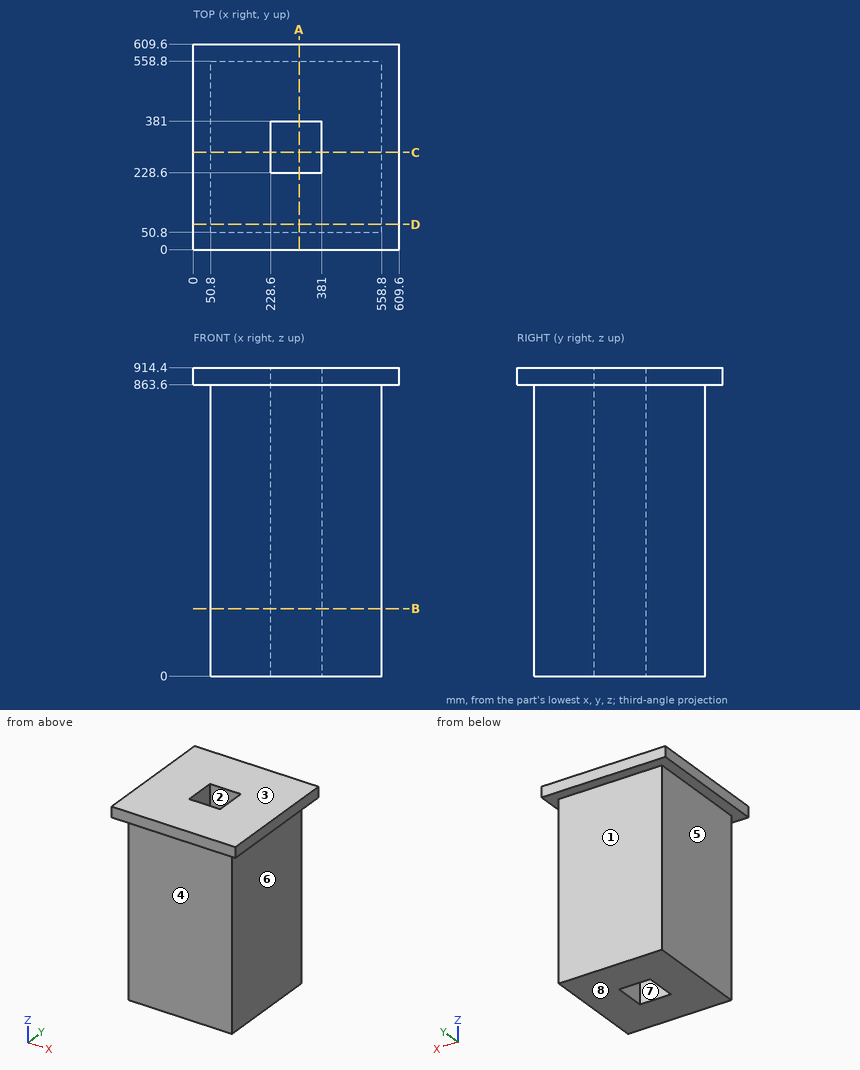
Print and shaded views of the part. All mm, measured from the part's lowest x, y and z. A direction names the side the tool comes from. Coordinates: 2 decimals unless noted, no trailing zeros. Order: outer loops, then holes, each group sorted by start corner. A loop starts at its lowest first (then second) coordinate and runs counter-clockwise, first axis right, second up. Notation, with made-up numbers: (26, 27) -> (47, 27) arc R12 cw to (47, 44) -> close; hole circle Ø8 at (6, 76). An arc over 180 degrees is marked (long way). Answer as a JSON object with one key per item and string values. Group by question number.
1) Pull direction X, two halves, no side cores. Call the marked faces 6, 7 and 8: +X half, -X half, draft (parallel to the pull), parting line (faces both ways), or undercut.
2) Flat gauge pins, fed straight in: pin 1 (3 mm diameter, centred on x = 88.5, y = 104, fed in from -Z); pin 2 (8 mm diameter, centred on y = 502, z = 176.5, fed in from +X); pin 3 (1.5 mm diameter, centred on x = 263.5, z = 226.5, fed in from +Y); pin 4 (5 mm diameter, centred on x = 315.5, z = 148, fed in from -Y). Where does each tip first touch, or does it go through?
3) Drill centre lines: L1, parallel to Y at x = 345, z = 298.5; L2, parallel to X at y = 139, z = 670. Where is each one in solid material? Low to high.
4) Cut at B-B, the plane z = 200. Write the cut outline in (x, y).
5) Cut at A-A, the plane x = 313.5. Write the cut outline in (y, z).
6) Cut at D-D, the plane y = 75. Write the cut outline in (x, z), then the cut area to 3 significant figures.
7) Which spindle directions (+Z, -Z, +X, -X, +Y, -Y) get a long thin tool onto all of the face, cutting with end or side? Do the marked faces 1, 2, 3, 4 and 5. Say none if no direction does.
Check values:
{
 "1": {"face 6": "+X half", "face 7": "undercut", "face 8": "draft"},
 "2": {"pin 1": "stops at z = 0", "pin 2": "stops at x = 558.8", "pin 3": "stops at y = 558.8", "pin 4": "stops at y = 50.8"},
 "3": {"L1": "y = 50.8 to 228.6, 381 to 558.8", "L2": "x = 50.8 to 558.8"},
 "4": {"outline": "(50.8, 50.8) -> (558.8, 50.8) -> (558.8, 558.8) -> (50.8, 558.8) -> close; hole (228.6, 228.6) -> (381, 228.6) -> (381, 381) -> (228.6, 381) -> close"},
 "5": {"outline": "(0, 863.6) -> (50.8, 863.6) -> (50.8, 0) -> (228.6, 0) -> (228.6, 914.4) -> (0, 914.4) -> close; (381, 0) -> (558.8, 0) -> (558.8, 863.6) -> (609.6, 863.6) -> (609.6, 914.4) -> (381, 914.4) -> close"},
 "6": {"outline": "(0, 863.6) -> (50.8, 863.6) -> (50.8, 0) -> (558.8, 0) -> (558.8, 863.6) -> (609.6, 863.6) -> (609.6, 914.4) -> (0, 914.4) -> close", "area": "470,000 mm²"},
 "7": {"face 1": "-Z, +X, -X, +Y", "face 2": "+Z, -Z", "face 3": "+Z, +X, -X, +Y, -Y", "face 4": "-Z, +X, -X, -Y", "face 5": "-Z, -X, +Y, -Y"}
}
